Can you work these out from the drawing? Everything is in mm from the part's minimum corner. Coordinates: 2 decimals unless noted, no trailing zeros. Order: outer loops, then holes, each group sorted by start corner. A loop starts at its lowest first (then second) coordinate and runs counter-clockwise, first axis right, second up. Notation, with made-up numbers: (34.5, -2) - (44.5, -2) arc R12 cw to (44.5, 6) - close; hole circle Ø10 at (56, 85). An arc over 180 degrees is marked (long way). Use a Markdown table: item, result. Add a question column.
(1) I want a section at D-D (x = 9.5). List the corners of the cut face in (y, z) for me.
(2) If I drill on L1, parallel to Z at x = 9.5, y = 3.55; L2, parallel to X at y = 5.75, z = 11.75; L3, parallel to Z at x = 72, y = 6, over which ranges is the centre line in solid material (lowest first)? Write a range as [from, to].
(3) For pin 1 Ø1 at (y, z) = (1, 15.5) entering from -X; pin 2 Ø9.5 at (x, z) = (72, 12.5) entering from -Y; pin 3 Ø10.5 at (x, z) = (34.5, 12.5) entering from -Y, each with a flat end and sliding along its axis, tell me the tip position at first contact or that it passes through.
(4) I want a section at A-A (x = 72). List the corners of the cut face in (y, z) for me.
(5) I want a section at B-B (z = 12.5). List the corners of the cut face in (x, y) for me.
(6) We'd pull the mould along X, two halves only. Please class the marked faces 1 and 2: pulls with the +X half, pulls with the -X half, needs draft (parallel to the pull), parting line crosses it, or undercut.
(7) I want a section at C-C (y = 3). List the corners of the cut face in (x, z) for me.
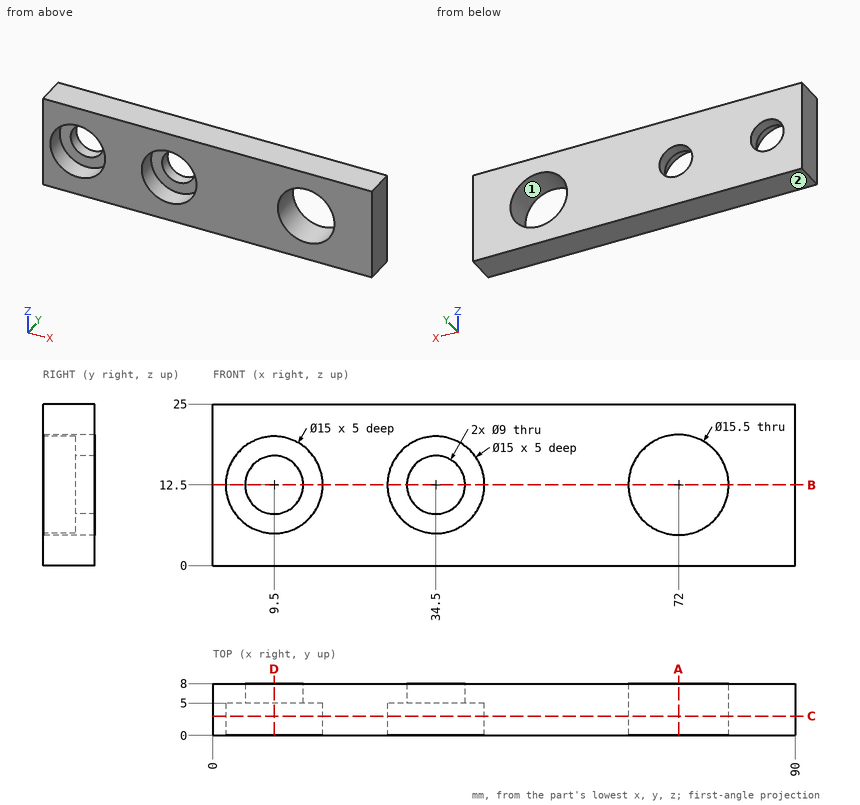
Answers follow:
| question | item | result |
|---|---|---|
| 1 | outline | (0, 0) - (8, 0) - (8, 8) - (5, 8) - (5, 5) - (0, 5) - close; (0, 20) - (5, 20) - (5, 17) - (8, 17) - (8, 25) - (0, 25) - close |
| 2 | L1 | z = [0, 5], [20, 25] |
| 2 | L2 | x = [0, 5.06], [13.94, 30.06], [38.94, 64.29], [79.71, 90] |
| 2 | L3 | z = [0, 4.75], [20.25, 25] |
| 3 | pin 1 | stops at x = 0 |
| 3 | pin 2 | passes through |
| 3 | pin 3 | stops at y = 5 |
| 4 | outline | (0, 0) - (8, 0) - (8, 4.75) - (0, 4.75) - close; (0, 20.25) - (8, 20.25) - (8, 25) - (0, 25) - close |
| 5 | outline | (0, 0) - (2, 0) - (2, 5) - (5, 5) - (5, 8) - (0, 8) - close; (14, 5) - (17, 5) - (17, 0) - (27, 0) - (27, 5) - (30, 5) - (30, 8) - (14, 8) - close; (39, 5) - (42, 5) - (42, 0) - (64.25, 0) - (64.25, 8) - (39, 8) - close; (79.75, 0) - (90, 0) - (90, 8) - (79.75, 8) - close |
| 6 | face 1 | undercut |
| 6 | face 2 | needs draft |
| 7 | outline | (0, 0) - (90, 0) - (90, 25) - (0, 25) - close; hole circle Ø15 at (9.5, 12.5); hole circle Ø15 at (34.5, 12.5); hole circle Ø15.5 at (72, 12.5) |
